Here's how the part is built. I have some questions about the finished solid (model axes, mm). Coordinates: 2 decimals unless noted, no trailing zeros. Loops run counter-clockwise (first coordinate to the right, second up) from the corner with the lowest first, then second, coordinate; pieces in that order, holes last. Notation, with made-up numbers: (29.25, 37.5) -> (65.25, 37.5) arc R26 ccw to (65.25, 71.5) -> close; hole circle Ø1 at (36.5, -7). An arc over 180 degrees is marked (long way). Answer as a JSON object with one key per item and string values. Group by question number.
1) I want a section at C-C (y = -785.6). Write out the boundary of the cut face in (x, z), then the cut area to 3 significant figures.
2) If we mould it in two halves opening along X, with no side actions, what happens to faces 1 (the cylindrical face through (-8.81, -786.64, -2174.31)), 2 (the flat face through (-15, -787, -2173)), 3 (the flat face through (-5.7, -788.115, -2173.4))? For each: +X half, -X half, draft (parallel to the pull), parting line (faces both ways), or undercut.
3) I want a section at A-A (x = -7.5). Write out the boundary of the cut face in (y, z), then the cut area to 3 significant figures.
4) I need wall thicknesses on probe 1 along Z at (x, y) = (-7.5, -786.6); probe 2 along Z at (x, y) = (-6, -786.7); probe 3 along X at (y, z) = (-787.4, -2173.5). Which ranges of each line are inside material? Lowest first, please. Write a range as [from, to].
5) I want a section at B-B (z = -2172.5). Write out the boundary of the cut face in (x, y).
```python
from build123d import *

# Parameters (mm, degrees)
SKETCH_1_W             = 15
SKETCH_1_H             = 3
EXTRUDE_1_DEPTH        = 15
HOLE_WIZARD_M4_1_D     = 3.3
HOLE_WIZARD_M4_1_DEPTH = 11.5
HOLE_WIZARD_M4_1_TIP   = 0.991420021


with BuildPart() as part:
    # 草图1 → 凸台-拉伸1 (new body)
    with BuildSketch(Plane.ZY):
        with Locations((-2173.305231444, -786.615322881)):
            Rectangle(SKETCH_1_W, SKETCH_1_H)
    extrude(amount=EXTRUDE_1_DEPTH)

    # M4 螺纹孔1
    with Locations(Plane(origin=(0, -785.115322881, 0), x_dir=(-1, 0, 0), z_dir=(0, 1, 0))):
        with Locations((7.5, -2173.305231444)):
            Hole(HOLE_WIZARD_M4_1_D / 2, depth=HOLE_WIZARD_M4_1_DEPTH)
            with Locations((0, 0, -(HOLE_WIZARD_M4_1_DEPTH + HOLE_WIZARD_M4_1_TIP / 2))):  # 118° drill point
                Cone(0, HOLE_WIZARD_M4_1_D / 2, HOLE_WIZARD_M4_1_TIP, mode=Mode.SUBTRACT)


solid = part.part
```
Determined:
{
 "1": {"outline": "(-15, -2180.81) -> (0, -2180.81) -> (0, -2165.81) -> (-15, -2165.81) -> close; hole circle Ø3.3 at (-7.5, -2173.31)", "area": "216 mm^2"},
 "2": {"face 1": "undercut", "face 2": "-X half", "face 3": "draft"},
 "3": {"outline": "(-788.12, -2180.81) -> (-785.12, -2180.81) -> (-785.12, -2174.96) -> (-788.12, -2174.96) -> close; (-788.12, -2171.66) -> (-785.12, -2171.66) -> (-785.12, -2165.81) -> (-788.12, -2165.81) -> close", "area": "35.1 mm^2"},
 "4": {"probe 1": "[-2180.81, -2174.96], [-2171.66, -2165.81]", "probe 2": "[-2180.81, -2173.99], [-2172.62, -2165.81]", "probe 3": "[-15, -9.14], [-5.86, 0]"},
 "5": {"outline": "(-15, -788.12) -> (-8.94, -788.12) -> (-8.94, -785.12) -> (-15, -785.12) -> close; (-6.06, -788.12) -> (0, -788.12) -> (0, -785.12) -> (-6.06, -785.12) -> close"}
}
